from build123d import *

# Parameters (mm, degrees)
SKETCH2_R                = 1.4
BOSS_EXTRUDE1_DEPTH      = 12
BOSS_EXTRUDE5_DEPTH      = 2
BOSS_EXTRUDE2_REACH      = 30.617
BOSS_EXTRUDE2_END_RADIUS = 86
SKETCH3_W                = 14
SKETCH3_H                = 14
SKETCH15_W               = 10
SKETCH15_H               = 10
SKETCH15_H_2             = 2
CUT_EXTRUDE1_DEPTH       = 12
SKETCH16_R               = 1.25
CUT_EXTRUDE2_DEPTH       = 27.55044426


with BuildPart() as part:
    # Sketch2 → Boss-Extrude1 (new body)
    with BuildSketch(Plane(origin=(0, 0, 0), x_dir=(1, 0, 0), z_dir=(0, 1, 0))):
        with BuildLine():
            ThreePointArc((10.49446819, 8.279873701), (0, 7.5), (-10.49446819, 8.279873701))
            ThreePointArc((-10.49446819, 8.279873701), (-19.020657749, 1.97082531), (-12.711609357, -6.555364249))
            ThreePointArc((-12.711609357, -6.555364249), (0, -7.5), (12.711609357, -6.555364249))
            ThreePointArc((12.711609357, -6.555364249), (19.020657749, 1.97082531), (10.49446819, 8.279873701))
        make_face()
        with Locations(Location((-11.603038774, 0.862254726, 0), (0, 0, 270))):
            Circle(SKETCH2_R, mode=Mode.SUBTRACT)
        with Locations(Location((11.603038774, 0.862254726, 0), (0, 0, 270))):
            Circle(SKETCH2_R, mode=Mode.SUBTRACT)
    extrude(amount=BOSS_EXTRUDE1_DEPTH)

    # Sketch14 → Boss-Extrude5 (add)
    with BuildSketch(Plane(origin=(0, 12, 0), x_dir=(1, 0, 0), z_dir=(0, 1, 0))):
        with BuildLine():
            ThreePointArc((-10.49446819, 8.279873701), (-13.158435282, 8.199198347), (-15.625987479, 7.192016469))
            ThreePointArc((-15.625987479, 7.192016469), (0, 5.5), (15.625987479, 7.192016469))
            ThreePointArc((15.625987479, 7.192016469), (13.158435282, 8.199198347), (10.49446819, 8.279873701))
            ThreePointArc((10.49446819, 8.279873701), (0, 7.5), (-10.49446819, 8.279873701))
        make_face()
        with BuildLine():
            ThreePointArc((17.605627343, -3.634291778), (0, -5.5), (-17.605627343, -3.634291778))
            ThreePointArc((-17.605627343, -3.634291778), (-15.446905606, -5.577829728), (-12.711609357, -6.555364249))
            ThreePointArc((-12.711609357, -6.555364249), (0, -7.5), (12.711609357, -6.555364249))
            ThreePointArc((12.711609357, -6.555364249), (15.446905606, -5.577829728), (17.605627343, -3.634291778))
        make_face()
    extrude(amount=BOSS_EXTRUDE5_DEPTH)

    # Boss-Extrude2: up to this cylinder (the profile starts outside it)
    boss_extrude2_end = Plane(origin=(0, 7, -78.5), z_dir=(0, -1, 0)) * Cylinder(BOSS_EXTRUDE2_END_RADIUS, 234.234, mode=Mode.PRIVATE)
    # Sketch3 → Boss-Extrude2 (add, up to the surface)
    with BuildSketch(Plane.XY.offset(7.7), mode=Mode.PRIVATE) as boss_extrude2_sk1:
        with Locations((0, 7)):
            Rectangle(SKETCH3_W, SKETCH3_H)
    boss_extrude2_tool1 = extrude(boss_extrude2_sk1.sketch, amount=-BOSS_EXTRUDE2_REACH, mode=Mode.PRIVATE) - boss_extrude2_end
    add(boss_extrude2_tool1.solids().sort_by_distance((0, 7, 7.7))[0])

    # Sketch15 → Cut-Extrude1 (cut)
    with BuildSketch(Plane.XY.offset(7.7)):
        with Locations((0, 7)):
            Rectangle(SKETCH15_W, SKETCH15_H)
        with Locations((0, 13)):
            Rectangle(SKETCH15_W, SKETCH15_H_2)
    extrude(amount=-CUT_EXTRUDE1_DEPTH, mode=Mode.SUBTRACT)

    # Sketch16 → Cut-Extrude2 (cut, through all)
    with BuildSketch(Plane.XY.offset(-4.3)):
        with Locations((0, 7)):
            Circle(SKETCH16_R)
    extrude(amount=-CUT_EXTRUDE2_DEPTH, mode=Mode.SUBTRACT)


solid = part.part
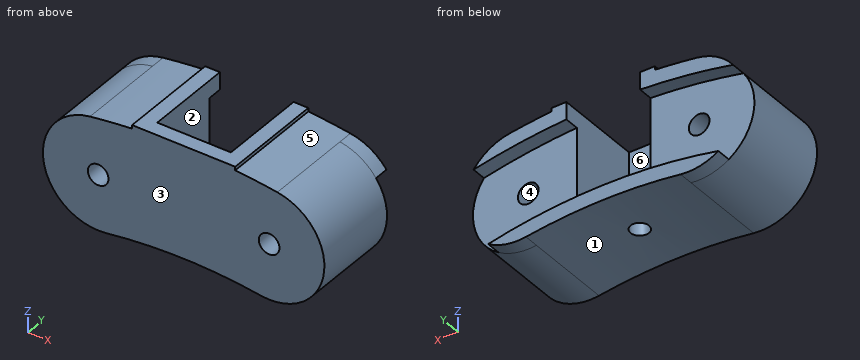
CAD build for the part. Positions are in the model's coordinates, mm. Face numbers are marked on the shaded views. A direction names the side the tool comes from. Give positions to 0.01 mm unless a question says otherwise; leave off trailing zeros. Loops run counter-clockwise (first coordinate to the right, second up) from the corner with the lowest first, then second, coordinate; pieces in that order, holes last. Notation, with made-up numbers: M 72.25,85.25 L 122.25,85.25 A13 ccw 122.25,108.25 Z; hole C 51.5,-13.5 d1. An arc over 180 degrees is marked long. Answer in a Markdown table with one row per item. Add a question column.
Item 1: Mould opens along X. For the marked faces 3, 4, 5 and 6 say: +X half, -X half, draft (parallel to the pull), parting line (faces both ways), or undercut.
Item 2: Tool access for the marked faces 1 and 2: list every direction of +Z, -Z, +X, -X, +Y, -Y with a clear straight run to the whole face (end or side of a thin tool).
Item 3: Band-saw the part on B-B on y = 7. Give the cut face in (x, z), then the cut area to 3 significant figures.
Item 4: Band-saw the part on C-C on y = 12.75. Give the cut face in (x, z).
Item 5: Band-saw the part on D-D on z = -0.25. Give the cut face in (x, y).
Item 6: Probe probe 1 along Y at (x, z) = (0, -5.9); probe 2 along Y at (x, z) = (-17, 0.5); probe 3 along Y at (x, z) = (2, 2.75). List the from-to ranges inside material, lowest first.
Item 7: Drop flat-ended pins along their axis: P1, Ø1.7, axis at x = 11.6, z = -0.86, coming from the +Y side; P2, Ø3, axis at x = 0, y = 7, coming from the +Z side; P3, Ø1.5, axis at x = -10.5, y = 12.5, coming from the -Z side; P4, Ø0.5, axis at y = 10, z = 7.5, coming from the -X side. Give the stop position or say it passes through.
Item 8: Band-saw the part on A-A on x = 0. Give the cut face in (y, z).
Reply:
| question | item | result |
|---|---|---|
| 1 | face 3 | draft |
| 1 | face 4 | undercut |
| 1 | face 5 | +X half |
| 1 | face 6 | undercut |
| 2 | face 1 | -Z, +Y, -Y |
| 2 | face 2 | +Z, +Y |
| 3 | outline | M -12.71,6.56 A7.5 ccw -10.49,-8.28 A71 cw -1.25,-7.51 L -1.25,-4.3 L -5,-4.3 L -5,7.7 L -7,7.7 L -7,7.21 A86 ccw Z; M 1.25,-7.51 A71 cw 10.49,-8.28 A7.5 ccw 12.71,6.56 A86 ccw 7,7.21 L 7,7.7 L 5,7.7 L 5,-4.3 L 1.25,-4.3 Z; hole C -11.6,-0.86 d2.8; hole C 11.6,-0.86 d2.8 |
| 3 | area | 390 mm^2 |
| 4 | outline | M -17.61,3.63 A84 cw -5,5.35 L -5,7.7 L -7,7.7 L -7,7.21 A86 ccw -12.71,6.56 A7.5 ccw Z; M -15.63,-7.19 A7.5 ccw -10.49,-8.28 A71 cw 10.49,-8.28 A7.5 ccw 15.63,-7.19 A73 ccw Z; M 5,5.35 A84 cw 17.61,3.63 A7.5 ccw 12.71,6.56 A86 ccw 7,7.21 L 7,7.7 L 5,7.7 Z |
| 5 | outline | M -19.08,0 L -12.86,0 L -12.86,12 L -19.08,12 Z; M -10.34,0 L 10.34,0 L 10.34,12 L 5,12 L 5,2 L -5,2 L -5,12 L -10.34,12 Z; M 12.86,0 L 19.08,0 L 19.08,12 L 12.86,12 Z |
| 6 | probe 1 | y = 0 to 5.75, 8.25 to 14 |
| 6 | probe 2 | y = 0 to 12 |
| 6 | probe 3 | y = 0 to 2 |
| 7 | P1 | passes through |
| 7 | P2 | stops at z = -4.3 |
| 7 | P3 | stops at z = -8.35 |
| 7 | P4 | stops at x = -7 |
| 8 | outline | M 0,-7.5 L 5.75,-7.5 L 5.75,-4.3 L 2,-4.3 L 2,7.7 L 0,7.7 Z; M 8.25,-7.5 L 14,-7.5 L 14,-5.5 L 12,-5.5 L 12,-4.3 L 8.25,-4.3 Z |
